Could you check a few things on this model? Use its own coordinates, in mm. Round coordinates to 2 decimals unless told otherwise and drop trailing zeros. Order: outer loops, then holes, each group sorted by start corner. A loop starts at its lowest first (then second) coordinate and runs counter-clockwise, first axis right, second up. Notation, with made-up numbers: (10.5, 74) - (58.5, 74) arc R7 cw to (58.5, 84) - close; hole circle Ø4 at (66.5, 23). An arc over 180 degrees is marked (long way). Return JSON: item names as keys, results as strings. Group by question number.
from build123d import *

# Parameters (mm, degrees)
SKETCH2_W               = 260
SKETCH2_H               = 100
BOSS_EXTRUDE1_DEPTH     = 4
SKETCH3_W               = 4.1
SKETCH3_H               = 20.2
CUT_EXTRUDE1_DEPTH      = 4
LPATTERN1_COUNT         = 3
LPATTERN1_PITCH         = 40
MIRROR1_COPY_1_SKETCH_W = 4.1
MIRROR1_COPY_1_SKETCH_H = 20.2
MIRROR1_COPY_1_DEPTH    = 4
MIRROR1_COPY_2_SKETCH_W = 4.1
MIRROR1_COPY_2_SKETCH_H = 20.2
MIRROR1_COPY_2_DEPTH    = 4
SKETCH4_W               = 20.2
SKETCH4_H               = 4.1
CUT_EXTRUDE2_DEPTH      = 4
LPATTERN2_COUNT         = 7
LPATTERN2_PITCH         = 40
MIRROR2_COPY_1_SKETCH_W = 20.2
MIRROR2_COPY_1_SKETCH_H = 4.1
MIRROR2_COPY_1_DEPTH    = 4
MIRROR2_COPY_2_SKETCH_W = 20.2
MIRROR2_COPY_2_SKETCH_H = 4.1
MIRROR2_COPY_2_DEPTH    = 4
MIRROR2_COPY_3_SKETCH_W = 20.2
MIRROR2_COPY_3_SKETCH_H = 4.1
MIRROR2_COPY_3_DEPTH    = 4
MIRROR2_COPY_4_SKETCH_W = 20.2
MIRROR2_COPY_4_SKETCH_H = 4.1
MIRROR2_COPY_4_DEPTH    = 4
MIRROR2_COPY_5_SKETCH_W = 20.2
MIRROR2_COPY_5_SKETCH_H = 4.1
MIRROR2_COPY_5_DEPTH    = 4
MIRROR2_COPY_6_SKETCH_W = 20.2
MIRROR2_COPY_6_SKETCH_H = 4.1
MIRROR2_COPY_6_DEPTH    = 4
SKETCH5_R               = 14
SKETCH5_R_2             = 1.75
CUT_EXTRUDE3_DEPTH      = 5


with BuildPart() as part:
    # Sketch2 → Boss-Extrude1 (new body)
    with BuildSketch(Plane.XY):
        Rectangle(SKETCH2_W, SKETCH2_H)
    extrude(amount=BOSS_EXTRUDE1_DEPTH)

    # Sketch3 → Cut-Extrude1 (cut)
    with BuildSketch(Plane.XY.offset(4)):
        with Locations((-127.95, -40)):
            Rectangle(SKETCH3_W, SKETCH3_H)
    cut_extrude1 = extrude(amount=-CUT_EXTRUDE1_DEPTH, mode=Mode.SUBTRACT)

    # LPattern1: Cut-Extrude1 ×3
    with Locations(*[(0, i * LPATTERN1_PITCH, 0) for i in range(1, LPATTERN1_COUNT)]):
        add(cut_extrude1, mode=Mode.SUBTRACT)

    # Mirror1: Cut-Extrude1 across plane
    add(cut_extrude1.mirror(Plane(origin=(0, 0, 0), x_dir=(0, 0, 1), z_dir=(1, 0, 0))), mode=Mode.SUBTRACT)

    # Mirror1 copy 1 sketch → Mirror1 copy 1 (cut)
    with BuildSketch(Plane(origin=(0, 40, 4), x_dir=(-1, 0, 0), z_dir=(0, 0, 1))):
        with Locations((-127.95, 40)):
            Rectangle(MIRROR1_COPY_1_SKETCH_W, MIRROR1_COPY_1_SKETCH_H)
    extrude(amount=-MIRROR1_COPY_1_DEPTH, mode=Mode.SUBTRACT)

    # Mirror1 copy 2 sketch → Mirror1 copy 2 (cut)
    with BuildSketch(Plane(origin=(0, 80, 4), x_dir=(-1, 0, 0), z_dir=(0, 0, 1))):
        with Locations((-127.95, 40)):
            Rectangle(MIRROR1_COPY_2_SKETCH_W, MIRROR1_COPY_2_SKETCH_H)
    extrude(amount=-MIRROR1_COPY_2_DEPTH, mode=Mode.SUBTRACT)

    # Sketch4 → Cut-Extrude2 (cut)
    with BuildSketch(Plane.XY.offset(4)):
        with Locations((-120, -47.95)):
            Rectangle(SKETCH4_W, SKETCH4_H)
    cut_extrude2 = extrude(amount=-CUT_EXTRUDE2_DEPTH, mode=Mode.SUBTRACT)

    # LPattern2: Cut-Extrude2 ×7
    with Locations(*[(i * LPATTERN2_PITCH, 0, 0) for i in range(1, LPATTERN2_COUNT)]):
        add(cut_extrude2, mode=Mode.SUBTRACT)

    # Mirror2: Cut-Extrude2 across plane
    add(cut_extrude2.mirror(Plane.ZX), mode=Mode.SUBTRACT)

    # Mirror2 copy 1 sketch → Mirror2 copy 1 (cut)
    with BuildSketch(Plane(origin=(40, 0, 4), x_dir=(1, 0, 0), z_dir=(0, 0, 1))):
        with Locations((-120, 47.95)):
            Rectangle(MIRROR2_COPY_1_SKETCH_W, MIRROR2_COPY_1_SKETCH_H)
    extrude(amount=-MIRROR2_COPY_1_DEPTH, mode=Mode.SUBTRACT)

    # Mirror2 copy 2 sketch → Mirror2 copy 2 (cut)
    with BuildSketch(Plane(origin=(80, 0, 4), x_dir=(1, 0, 0), z_dir=(0, 0, 1))):
        with Locations((-120, 47.95)):
            Rectangle(MIRROR2_COPY_2_SKETCH_W, MIRROR2_COPY_2_SKETCH_H)
    extrude(amount=-MIRROR2_COPY_2_DEPTH, mode=Mode.SUBTRACT)

    # Mirror2 copy 3 sketch → Mirror2 copy 3 (cut)
    with BuildSketch(Plane(origin=(120, 0, 4), x_dir=(1, 0, 0), z_dir=(0, 0, 1))):
        with Locations((-120, 47.95)):
            Rectangle(MIRROR2_COPY_3_SKETCH_W, MIRROR2_COPY_3_SKETCH_H)
    extrude(amount=-MIRROR2_COPY_3_DEPTH, mode=Mode.SUBTRACT)

    # Mirror2 copy 4 sketch → Mirror2 copy 4 (cut)
    with BuildSketch(Plane(origin=(160, 0, 4), x_dir=(1, 0, 0), z_dir=(0, 0, 1))):
        with Locations((-120, 47.95)):
            Rectangle(MIRROR2_COPY_4_SKETCH_W, MIRROR2_COPY_4_SKETCH_H)
    extrude(amount=-MIRROR2_COPY_4_DEPTH, mode=Mode.SUBTRACT)

    # Mirror2 copy 5 sketch → Mirror2 copy 5 (cut)
    with BuildSketch(Plane(origin=(200, 0, 4), x_dir=(1, 0, 0), z_dir=(0, 0, 1))):
        with Locations((-120, 47.95)):
            Rectangle(MIRROR2_COPY_5_SKETCH_W, MIRROR2_COPY_5_SKETCH_H)
    extrude(amount=-MIRROR2_COPY_5_DEPTH, mode=Mode.SUBTRACT)

    # Mirror2 copy 6 sketch → Mirror2 copy 6 (cut)
    with BuildSketch(Plane(origin=(240, 0, 4), x_dir=(1, 0, 0), z_dir=(0, 0, 1))):
        with Locations((-120, 47.95)):
            Rectangle(MIRROR2_COPY_6_SKETCH_W, MIRROR2_COPY_6_SKETCH_H)
    extrude(amount=-MIRROR2_COPY_6_DEPTH, mode=Mode.SUBTRACT)

    # Sketch5 → Cut-Extrude3 (cut, through all)
    with BuildSketch(Plane.XY.offset(4)):
        with Locations((-100, -15)):
            Circle(SKETCH5_R)
        with Locations((-111.5, -3.5)):
            Circle(SKETCH5_R_2)
        with Locations((-88.5, -3.5)):
            Circle(SKETCH5_R_2)
        with Locations((-111.5, -26.5)):
            Circle(SKETCH5_R_2)
        with Locations((-88.5, -26.5)):
            Circle(SKETCH5_R_2)
    extrude(amount=-CUT_EXTRUDE3_DEPTH, mode=Mode.SUBTRACT)


solid = part.part
1) I want a section at D-D, the plane x = -7. List the corners of the cut face in (y, z) for me, plus the area to 3 significant figures.
2) I want a section at A-A, the plane x = -100. List the corners of the cut face in (y, z) for me.
3) If I drill on line 1 along X through (y, z) = (-10.5, 3.55); line 2 along Y through (x, z) = (-100.5, 1.45); line 3 along Y through (x, z) = (-88.5, 2.9), over which ranges is the centre line in solid material (lowest first)? Write a range as from..to.
4) We'd pull the mould along X, two halves only. Please class faces 1 (the flat face through (-2, 1, 0)), 2 (the cylindrical face through (-87.068, -20.362, 2.028)): +X half, -X half, draft (parallel to the pull), parting line (faces both ways), or undercut.
5) Will these pins go through, and if not, where does the flat tip stop? pin 1 (2 mm diameter, centred on y = -49, z = 1.5, fed in from -X); pin 2 (25 mm diameter, centred on x = -100, y = -15, fed in from +Z); pin 3 (1.2 mm diameter, centred on y = 48.5, z = 2, fed in from +X); pin 4 (1.2 mm diameter, centred on y = -2, z = 1.5, fed in from +X).
6) I want a section at B-B, the plane y = -15. List the corners of the cut face in (x, z) for me.
7) I want a section at C-C, the plane z = 1.15. Give the number of separate pieces and of enclosed holes in the cut face, plus the area to 3 significant figures.
Outcome:
{
 "1": {"outline": "(-45.9, 0) - (45.9, 0) - (45.9, 4) - (-45.9, 4) - close", "area": "367 mm^2"},
 "2": {"outline": "(-50, 0) - (-29, 0) - (-29, 4) - (-50, 4) - close; (-1, 0) - (50, 0) - (50, 4) - (-1, 4) - close"},
 "3": {"line 1": "-130..-113.26, -86.74..130", "line 2": "-50..-28.99, -1.01..50", "line 3": "-45.9..-28.25, -24.75..-22.98, -7.02..-5.25, -1.75..45.9"},
 "4": {"face 1": "draft", "face 2": "undercut"},
 "5": {"pin 1": "x = -109.9", "pin 2": "through", "pin 3": "x = 109.9", "pin 4": "x = 125.9"},
 "6": {"outline": "(-130, 0) - (-114, 0) - (-114, 4) - (-130, 4) - close; (-86, 0) - (130, 0) - (130, 4) - (-86, 4) - close"},
 "7": {"separate pieces": "1", "enclosed holes": "5", "area": "23,800 mm^2"}
}
